Here's how the part is built. I have some questions about the finished solid (model axes, mm). Face numbers are marked on the shaded views. A direction names the side the tool comes from. Round coordinates to 2 decimals unless told otherwise and drop trailing zeros. Loops run counter-clockwise (first coordinate to the right, second up) from the corner with the lowest first, then second, coordinate; pieces in that order, holes last. Notation, with made-up numbers: (4, -29.5) -> (56, -29.5) arc R28 ccw to (56, -8.5) -> close; hole circle Ø6 at (19.5, 87.25). An arc over 180 degrees is marked (long way). Use one line per item in the form item = value. Start each with the question number.
Item 1: If we section it at C-C (z = 20): Write out the boundary of the cut face in (x, y).
Item 2: I'm going to push flat-ended pins straight in: pin 1 Ø1.5 at (y, z) = (18, 18) entering from +X; pin 2 Ø3 at (y, z) = (7, 16.5) entering from -X; pin 3 Ø4 at (x, y) = (4.5, 4.5) entering from +Z. Where does each tip first touch, or does it pass through?
Item 3: Thinking about a two-plate mould opening in Y: for the marked faces 1, 2 and 3, which applies, released by +Y, released by -Y, zero draft, split by the parting line, or undercut?
Item 4: If we section it at A-A (y = 9.25): Write out the boundary of the cut face in (x, z).
Item 5: If we section it at B-B (z = 10.5): Write out the boundary of the cut face in (x, y), then the cut area to 3 significant figures.
Item 6: For the marked faces 4, 5 and 6, which set-ups out of +Z, -Z, +X, -X, +Y, -Y let a thin tool reach every point of the face, with its end or its side?
Item 7: If I drill on L1, parallel to Y at x = 11.5, z = 10.75; L2, parallel to Z at x = 15.75, y = 6.5; L3, parallel to Z at x = 11.75, y = 19.75, over which ranges is the centre line in solid material (lowest first)? Write a range as [from, to].
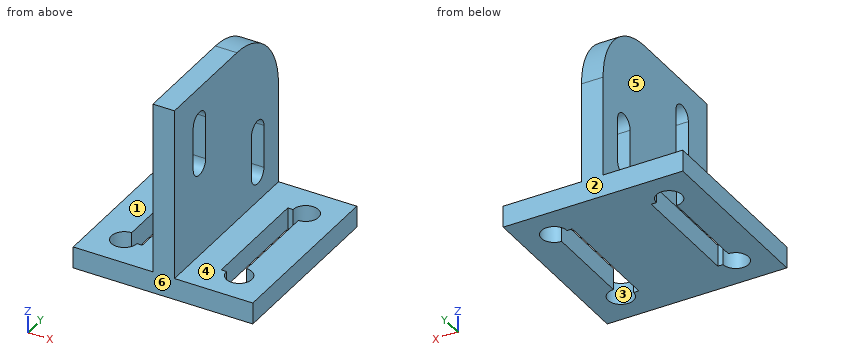
```python
from build123d import *

# Parameters (mm, degrees)
ESQUISSE1_W             = 25
ESQUISSE1_H             = 25
BOSS_EXTRU_1_DEPTH      = 3
ESQUISSE4_R             = 1.775
ESQUISSE4_W             = 2.5
ESQUISSE4_H             = 16
ENL_V_MAT_EXTRU_1_DEPTH = 10
ESQUISSE5_W             = 3
ESQUISSE5_H             = 25
BOSS_EXTRU_3_DEPTH      = 24
ENL_V_MAT_EXTRU_2_DEPTH = 10
CONG_1_R                = 10


with BuildPart() as part:
    # Esquisse1 → Boss.-Extru.1 (new body)
    with BuildSketch(Plane.XY):
        with Locations((12.5, 12.5)):
            Rectangle(ESQUISSE1_W, ESQUISSE1_H)
    extrude(amount=BOSS_EXTRU_1_DEPTH)

    # Esquisse4 → Enlèv. mat.-Extru.1 (cut)
    with BuildSketch(Plane(origin=(0, 0, 0), x_dir=(-1, 0, 0), z_dir=(0, 0, -1))):
        with BuildLine():
            Line((-20.5, 6.275), (-20.5, 4.5))
            Line((-20.5, 4.5), (-18.725, 4.5))
            ThreePointArc((-18.725, 4.5), (-19.244885463, 5.755114537), (-20.5, 6.275))
        make_face()
        with BuildLine():
            Line((-18.725, 4.5), (-20.5, 4.5))
            Line((-20.5, 4.5), (-20.5, 6.275))
            ThreePointArc((-20.5, 6.275), (-21.755114537, 3.244885463), (-18.725, 4.5))
        make_face()
        with Locations((-20.5, 20.5)):
            Circle(ESQUISSE4_R)
        with Locations((-20.5, 4.5)):
            Circle(ESQUISSE4_R)
        with Locations((-19.25, 12.5)):
            Rectangle(ESQUISSE4_W, ESQUISSE4_H)
        with BuildLine():
            ThreePointArc((-18.725, 20.5), (-21.755114537, 21.755114537), (-20.5, 18.725))
            Line((-20.5, 18.725), (-20.5, 20.5))
            Line((-20.5, 20.5), (-18.725, 20.5))
        make_face()
        with BuildLine():
            Line((-20.5, 20.5), (-20.5, 18.725))
            ThreePointArc((-20.5, 18.725), (-19.244885463, 19.244885463), (-18.725, 20.5))
            Line((-18.725, 20.5), (-20.5, 20.5))
        make_face()
        with BuildLine():
            Line((-4.5, 18.725), (-4.5, 20.5))
            Line((-4.5, 20.5), (-6.275, 20.5))
            ThreePointArc((-6.275, 20.5), (-5.755114537, 19.244885463), (-4.5, 18.725))
        make_face()
        with BuildLine():
            Line((-6.275, 20.5), (-4.5, 20.5))
            Line((-4.5, 20.5), (-4.5, 18.725))
            ThreePointArc((-4.5, 18.725), (-3.244885463, 19.244885463), (-2.725, 20.5))
            ThreePointArc((-2.725, 20.5), (-4.5, 22.275), (-6.275, 20.5))
        make_face()
        with Locations((-4.5, 4.5)):
            Circle(ESQUISSE4_R)
        with Locations((-4.5, 20.5)):
            Circle(ESQUISSE4_R)
        with Locations((-5.75, 12.5)):
            Rectangle(ESQUISSE4_W, ESQUISSE4_H)
        with BuildLine():
            ThreePointArc((-2.725, 4.5), (-3.244885463, 5.755114537), (-4.5, 6.275))
            Line((-4.5, 6.275), (-4.5, 4.5))
            Line((-4.5, 4.5), (-6.275, 4.5))
            ThreePointArc((-6.275, 4.5), (-4.5, 2.725), (-2.725, 4.5))
        make_face()
        with BuildLine():
            Line((-4.5, 4.5), (-4.5, 6.275))
            ThreePointArc((-4.5, 6.275), (-5.755114537, 5.755114537), (-6.275, 4.5))
            Line((-6.275, 4.5), (-4.5, 4.5))
        make_face()
    extrude(amount=-ENL_V_MAT_EXTRU_1_DEPTH, mode=Mode.SUBTRACT)

    # Esquisse5 → Boss.-Extru.3 (add)
    with BuildSketch(Plane.XY.offset(3)):
        with Locations((12.6, 12.5)):
            Rectangle(ESQUISSE5_W, ESQUISSE5_H)
    extrude(amount=BOSS_EXTRU_3_DEPTH)

    # Esquisse6 → Enlèv. mat.-Extru.2 (cut)
    with BuildSketch(Plane(origin=(14.1, 0, 0), x_dir=(0, 0, -1), z_dir=(1, 0, 0))):
        with BuildLine():
            Line((-22, 7.5), (-16, 7.5))
            ThreePointArc((-16, 7.5), (-14.5, 6), (-16, 4.5))
            Line((-16, 4.5), (-22, 4.5))
            ThreePointArc((-22, 4.5), (-23.5, 6), (-22, 7.5))
        make_face()
        with BuildLine():
            Line((-7, 18.5), (-13, 18.5))
            ThreePointArc((-13, 18.5), (-14.5, 20), (-13, 21.5))
            Line((-13, 21.5), (-7, 21.5))
            ThreePointArc((-7, 21.5), (-5.5, 20), (-7, 18.5))
        make_face()
    extrude(amount=-ENL_V_MAT_EXTRU_2_DEPTH, mode=Mode.SUBTRACT)

    # Congé1
    cong_1_edges = [part.edges().sort_by_distance(p)[0] for p in [
        (12.6, 25, 27),
    ]]
    fillet(cong_1_edges, radius=CONG_1_R)


solid = part.part
```
Values found:
q1.outline = (11.1, 0) -> (14.1, 0) -> (14.1, 4.5) -> (11.1, 4.5) -> close; (11.1, 7.5) -> (14.1, 7.5) -> (14.1, 24.54) -> (11.1, 24.54) -> close
q2.pin_1 = 14.1
q2.pin_2 = 11.1
q2.pin_3 = 3
q3.face_1 = zero draft
q3.face_2 = released by +Y
q3.face_3 = undercut
q4.outline = (0, 0) -> (4.5, 0) -> (4.5, 3) -> (0, 3) -> close; (7, 0) -> (18, 0) -> (18, 3) -> (14.1, 3) -> (14.1, 27) -> (11.1, 27) -> (11.1, 3) -> (7, 3) -> close; (20.5, 0) -> (25, 0) -> (25, 3) -> (20.5, 3) -> close
q5.outline = (11.1, 0) -> (14.1, 0) -> (14.1, 18.5) -> (11.1, 18.5) -> close; (11.1, 21.5) -> (14.1, 21.5) -> (14.1, 25) -> (11.1, 25) -> close
q5.area = 66.0 mm2
q6.face_4 = +Z, +X, +Y, -Y
q6.face_5 = +Z, -X, +Y, -Y
q6.face_6 = +Z, -Z, +X, -X, -Y
q7.L1 = [0, 18.5], [21.5, 25]
q7.L2 = [0, 3]
q7.L3 = [0, 5.52], [14.48, 25.8]
